Work out the finished part from the listing and answer in its coordinate system (mm). Face numbers are marked on the shaded views. Give positions to 0.01 mm unless a question says otherwise; leave off trailing zeros. Write each loop counter-clockwise with the first axis right and the second up, starting at its lowest first coordinate (ties: lowest second). Pieces come first, ordered by that corner, then holes.
1) Given pin 1 Ø1 at (x, z) = (2.5, -13.5) entering from -Y; pin 2 Ø1.8 at (y, z) = (1, -1.5) entering from -X, each flat-ended and moving along its own axis, determine where each tip first touches the part or whether it passes through.
2) Find section A-A (x = -2). Determine the outline of the cut face in (y, z).
3) Straight lines are drawn through the part: probe 1 along Z at (x, y) = (17, 0.5); probe 2 along Z at (x, y) = (9.5, -0.25); probe 3 along Y at (x, z) = (3, 8). For each, find the intervals that lie inside material, in ascending order.
4) Find section B-B (y = -1.5). Determine the outline of the cut face in (x, z), plus the area to 3 significant figures.
5) Find section C-C (z = -1.5). Determine the outline of the cut face in (x, y), plus the area to 3 significant figures.
6) Determine the mould class of the marked faces 1, 2 and 3 for opening direction Z: pulls with the +Z half, pulls with the -Z half, needs draft (parallel to the pull), parting line crosses it, or undercut.
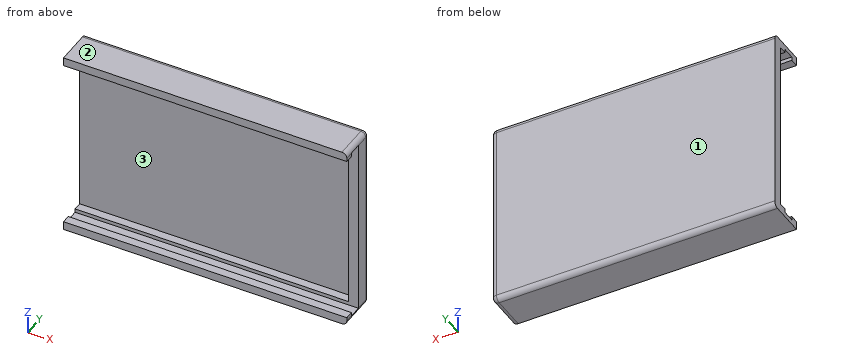
```python
from build123d import *

# Parameters (mm, degrees)
SKETCH1_W           = 56.896
SKETCH1_H           = 38.1
BOSS_EXTRUDE1_DEPTH = 3.937
CUT_EXTRUDE1_DEPTH  = 61.12950428
FILLET1_R           = 1
SKETCH3_W           = 34.767886748
SKETCH3_H           = 4.174
CUT_EXTRUDE2_DEPTH  = 54.896


with BuildPart() as part:
    # Sketch1 → Boss-Extrude1 (new, symmetric)
    with BuildSketch(Plane(origin=(0, 0, 0), x_dir=(1, 0, 0), z_dir=(0, 1, 0))):
        Rectangle(SKETCH1_W, SKETCH1_H)
    extrude(amount=BOSS_EXTRUDE1_DEPTH, both=True)

    # Sketch2 → Cut-Extrude1 (cut, through all)
    with BuildSketch(Plane(origin=(28.448, 0, 0), x_dir=(0, 0, -1), z_dir=(1, 0, 0))):
        Polygon((18.0975, -2.237), (18.0975, 0.263), (17.492836072, 0.263), (-17.492836072, 0.263), (-18.0975, 0.263), (-18.0975, -2.237), (-17.35, -2.237), (-17.35, -3.937), (17.35, -3.937), (17.35, -2.237), align=None)
    extrude(amount=-CUT_EXTRUDE1_DEPTH, mode=Mode.SUBTRACT)

    # Fillet1
    # the kernel refuses this fillet: 1 mm, written as the material it takes off along each edge
    with BuildSketch(Plane(origin=(27.448, 2.937, -18.05), x_dir=(1, 0, 0), z_dir=(0, 0, -1))) as fillet1_piece_1_section:
        Polygon((0, 0), (FILLET1_R, 0), (FILLET1_R, -FILLET1_R), (0, -FILLET1_R), align=None)
    fillet1_piece_1 = extrude(amount=FILLET1_R, mode=Mode.PRIVATE)
    fillet1_piece_1 = fillet1_piece_1 - Plane(origin=(27.448, 2.937, -18.05), x_dir=(-0.7071067811865475, -0.7071067811865475, 0), z_dir=(0, 0, -1)) * Sphere(FILLET1_R, mode=Mode.PRIVATE)
    add(fillet1_piece_1, mode=Mode.SUBTRACT)
    with BuildSketch(Plane(origin=(27.448, 2.937, 18.05), x_dir=(0, 1, 0), z_dir=(1, 0, 0))) as fillet1_piece_2_section:
        Polygon((0, 0), (FILLET1_R, 0), (FILLET1_R, FILLET1_R), (0, FILLET1_R), align=None)
    fillet1_piece_2 = extrude(amount=FILLET1_R, mode=Mode.PRIVATE)
    fillet1_piece_2 = fillet1_piece_2 - Plane(origin=(27.448, 2.937, 18.05), x_dir=(0, -0.7071067811865475, -0.7071067811865475), z_dir=(1, 0, 0)) * Sphere(FILLET1_R, mode=Mode.PRIVATE)
    add(fillet1_piece_2, mode=Mode.SUBTRACT)
    with BuildSketch(Plane(origin=(-30.948, 3.937, -19.05), x_dir=(0, -1, 0), z_dir=(1, 0, 0))) as fillet1_piece_3:
        with BuildLine():
            CenterArc((FILLET1_R, -FILLET1_R), FILLET1_R, 90, 90)
            Line((0, -FILLET1_R), (0, 0))
            Line((0, 0), (FILLET1_R, 0))
        make_face()
    extrude(amount=58.396, mode=Mode.SUBTRACT)
    with BuildSketch(Plane(origin=(28.448, 3.937, -18.05), x_dir=(0, -1, 0), z_dir=(0, 0, 1))) as fillet1_piece_4:
        with BuildLine():
            CenterArc((FILLET1_R, -FILLET1_R), FILLET1_R, 90, 90)
            Line((0, -FILLET1_R), (0, 0))
            Line((0, 0), (FILLET1_R, 0))
        make_face()
    extrude(amount=36.1, mode=Mode.SUBTRACT)
    with BuildSketch(Plane(origin=(27.448, 3.937, 19.05), x_dir=(0, 0, -1), z_dir=(-1, 0, 0))) as fillet1_piece_5:
        with BuildLine():
            CenterArc((FILLET1_R, FILLET1_R), FILLET1_R, 180, 90)
            Line((0, FILLET1_R), (0, 0))
            Line((0, 0), (FILLET1_R, 0))
        make_face()
    extrude(amount=58.396, mode=Mode.SUBTRACT)
    with BuildSketch(Plane(origin=(28.448, 2.937, -19.05), x_dir=(-1, 0, 0), z_dir=(0, -1, 0)), Plane(origin=(28.448, 2.937, 19.05), x_dir=(0, 0, -1), z_dir=(0, -1, 0))) as fillet1_piece_6:
        with BuildLine():
            CenterArc((FILLET1_R, -FILLET1_R), FILLET1_R, 90, 90)
            Line((0, -FILLET1_R), (0, 0))
            Line((0, 0), (FILLET1_R, 0))
        make_face()
    extrude(amount=9.374, mode=Mode.SUBTRACT)

    # Sketch3 → Cut-Extrude2 (cut)
    with BuildSketch(Plane.ZY.offset(28.448)):
        with Locations((0.033943374, -0.15)):
            Rectangle(SKETCH3_W, SKETCH3_H)
    extrude(amount=-CUT_EXTRUDE2_DEPTH, mode=Mode.SUBTRACT)


solid = part.part
```
Results:
1. pin 1: stops at y = 1.94
1. pin 2: stops at x = 26.45
2. outline: (-3.94, -19.05) - (2.94, -19.05) arc R1 ccw to (3.94, -18.05) - (3.94, 18.05) arc R1 ccw to (2.94, 19.05) - (-3.94, 19.05) - (-3.94, 17.35) - (-2.24, 17.35) - (-2.24, 18.1) - (0.26, 18.1) - (0.26, 17.42) - (1.94, 17.42) - (1.94, -17.35) - (0.26, -17.35) - (0.26, -18.1) - (-2.24, -18.1) - (-2.24, -17.35) - (-3.94, -17.35) - close
3. probe 1: z = -19.05 to -17.35, 17.42 to 19.05
3. probe 2: z = -19.05 to -18.1, 18.1 to 19.05
3. probe 3: y = 1.94 to 3.94
4. outline: (-28.45, -19.05) - (27.45, -19.05) arc R1 ccw to (28.45, -18.1) - (-28.45, -18.1) - close; (-28.45, 18.1) - (28.45, 18.1) arc R1 ccw to (27.45, 19.05) - (-28.45, 19.05) - close
4. area: 108 mm2
5. outline: (-28.45, 1.94) - (26.45, 1.94) - (26.45, 0.26) - (28.45, 0.26) - (28.45, 2.94) arc R1 ccw to (27.45, 3.94) - (-28.45, 3.94) - close
5. area: 117 mm2
6. face 1: needs draft
6. face 2: pulls with the +Z half
6. face 3: undercut
